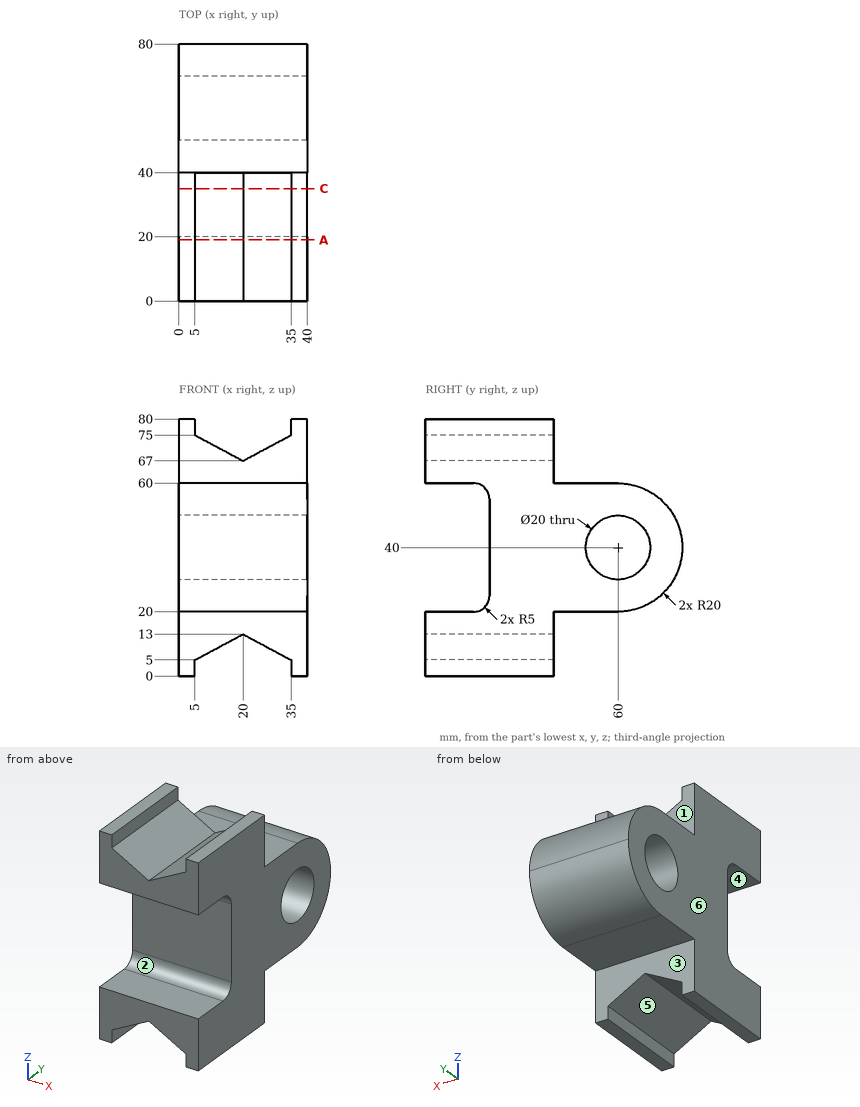
Job drawing, mm, ordinate dimensions from the low corner. One solid piece. A direction names the side the tool comes from. Give positions to 0.01 mm unless a question says otherwise; leave off trailing zeros. Write each loop counter-clockwise with the first axis right and the second up, starting at its lowest first coordinate (ties: lowest second). Pieces come first, ordered by that corner, then holes. Notation, with made-up numbers: (-5, 53) - (21, 53) arc R24 ccw to (21, 74) - close; hole circle Ø4 at (-22.75, 84.25). An arc over 180 degrees is marked (long way). Use one line per item in the form item = value. Start each with the question number.
1. Probe line 1 (Z direction, x = 10, y = 60); line 2 (Y direction, x = 17.5, z = 40); line 3 (Z direction, x = 36, y = 53). List the from-to ranges inside material, lowest first. Write a range as [from, to].
2. Band-saw the part on A-A on y = 19. Write the cut outline in (x, z), plus the area to 3 significant figures.
3. Two-plate mould, pull along X, no slides. Class the marked faces 4, 5 and 6: released by +X, released by -X, zero draft, split by the parting line, or undercut.
4. 3-axis set-ups, long thin cutter, end or side, ignore diameter. For the marked faces 1, 2 and 3: which of +Z, -Z, +X, -X, +Y, -Y reach the whole face in a straight line?
5. Band-saw the part on C-C on y = 35. Write the cut outline in (x, z), plus the area to 3 significant figures.
6. Drop flat-ended pins along their axis: pin 1 Ø5 at (x, y) = (28, 51) entering from +Z; pin 2 Ø10 at (x, y) = (13.5, 49.5) entering from -Z; pin 3 Ø12 at (x, y) = (19.5, 6.5) entering from +Z; pin 4 Ø18 at (y, z) = (60, 40) entering from +X. Give the stop position or say it passes through.
Conclusion:
q1.line_1 = [20, 30], [50, 60]
q1.line_2 = [20, 50], [70, 80]
q1.line_3 = [20, 32.86], [47.14, 60]
q2.outline = (0, 0) - (5, 0) - (5, 5) - (20, 13) - (35, 5) - (35, 0) - (40, 0) - (40, 22) - (0, 22) - close; (0, 58) - (40, 58) - (40, 80) - (35, 80) - (35, 75) - (20, 67) - (5, 75) - (5, 80) - (0, 80) - close
q2.area = 1,220 mm²
q3.face_4 = zero draft
q3.face_5 = undercut
q3.face_6 = released by -X
q4.face_1 = +Z, +X, -X, +Y
q4.face_2 = +X, -X, -Y
q4.face_3 = -Z, +X, -X, +Y
q5.outline = (0, 0) - (5, 0) - (5, 5) - (20, 13) - (35, 5) - (35, 0) - (40, 0) - (40, 80) - (35, 80) - (35, 75) - (20, 67) - (5, 75) - (5, 80) - (0, 80) - close
q5.area = 2,660 mm²
q6.pin_1 = 60
q6.pin_2 = 20
q6.pin_3 = 70.47
q6.pin_4 = through
